Answer from the drawing. Dimensions are ordinates in mm from the lowest x, y and z of the part. A direction names the side the tool comes from. Coordinates: 2 decimals unless noted, no trailing zeros. Order: outer loops, then holes, each group sorted by start corner. A loop starts at its lowest first (then second) coordinate and runs counter-clockwise, first axis right, second up. Notation, with made-up numbers: (-31, 62) - (-18, 62) arc R27 cw to (-18, 96) - close; hole circle Ø2 at (-12.5, -5.5). An arc over 180 degrees is marked (long way). One line per item, written item: value. Start each with the question number.
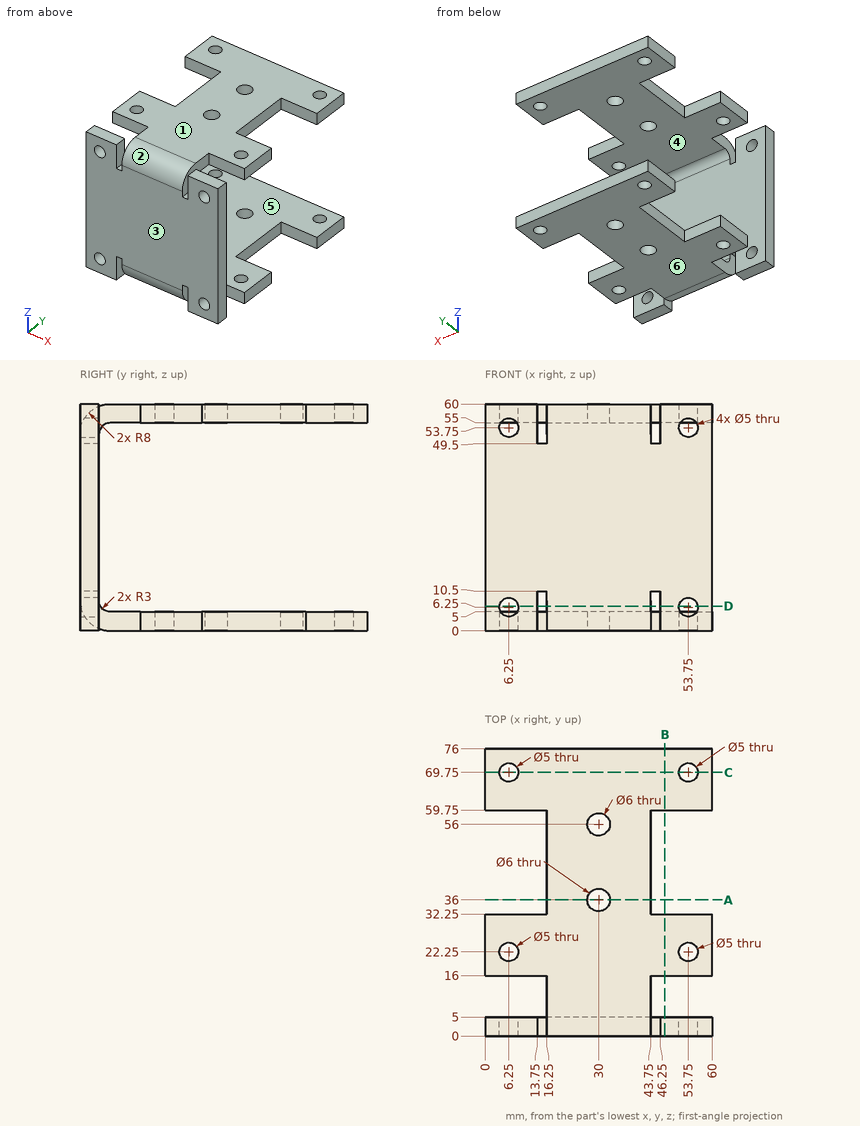
(1) The part is cut by section B-B on x = 47.5. Determine the outline of the cut face in (y, z).
(2) For the marked faces 1 and 2, determine the directions among +Z, -Z, +X, -X, +Y, -Y from which every point of the face is accessible in a straight line to the end or side of a thin tool.
(3) Flat-ended cylindrical pins translate along their axes: pin 1 Ø8 at (x, z) = (22, 31.5) entering from +Y; pin 2 Ø1.2 at (x, y) = (15.5, 2) entering from -Z; pin 3 Ø2.5 at (y, z) = (43.5, 58.5) entering from +X. Find the tip coordinate at first contact, or state that the pin passes through.
(4) For a pull along Z with two mould halves and no side action, classify the marked faces 3, 4, 5 and 6 as pulls with the +Z half, pulls with the -Z half, needs draft (parallel to the pull), parting line crosses it, or undercut.
(5) The part is cut by section D-D on z = 6.5. Determine the outline of the cut face in (x, y), plus the area to 3 significant figures.
(6) The part is cut by section A-A on y = 36. Determine the outline of the cut face in (x, z).
(7) Consider probe 1 along Z at (x, y) = (6, 3); probe 2 along Y at (x, z) = (6.25, 56.8); probe 3 along Y at (x, z) = (53, 57). Determine where each line is inside the solid, lowest interval first.
(8) The part is cut by section C-C on y = 69.75. Determine the outline of the cut face in (x, z), plus the area to 3 significant figures.
Completed:
1. outline: (0, 0) - (5, 0) - (5, 60) - (0, 60) - close; (16, 0) - (32.25, 0) - (32.25, 5) - (16, 5) - close; (16, 55) - (32.25, 55) - (32.25, 60) - (16, 60) - close; (59.75, 0) - (76, 0) - (76, 5) - (59.75, 5) - close; (59.75, 55) - (76, 55) - (76, 60) - (59.75, 60) - close
2. face 1: +Z, +X, -X, +Y, -Y
2. face 2: +Z, -Y
3. pin 1: stops at y = 5
3. pin 2: stops at z = 10.5
3. pin 3: stops at x = 43.75
4. face 3: needs draft
4. face 4: undercut
4. face 5: undercut
4. face 6: pulls with the -Z half
5. outline: (0, 0) - (3.76, 0) - (3.76, 5) - (0, 5) - close; (8.74, 0) - (13.75, 0) - (13.75, 5) - (8.74, 5) - close; (16.25, 0.14) - (43.75, 0.14) - (43.75, 5.4) - (16.25, 5.4) - close; (46.25, 0) - (51.26, 0) - (51.26, 5) - (46.25, 5) - close; (56.24, 0) - (60, 0) - (60, 5) - (56.24, 5) - close
5. area: 232 mm2
6. outline: (16.25, 0) - (27, 0) - (27, 5) - (16.25, 5) - close; (16.25, 55) - (27, 55) - (27, 60) - (16.25, 60) - close; (33, 0) - (43.75, 0) - (43.75, 5) - (33, 5) - close; (33, 55) - (43.75, 55) - (43.75, 60) - (33, 60) - close
7. probe 1: z = 0 to 3.76, 8.74 to 51.26, 56.24 to 60
7. probe 2: y = 0 to 5, 16 to 19.75, 24.75 to 32.25, 59.75 to 67.25, 72.25 to 76
7. probe 3: y = 0 to 5, 16 to 19.87, 24.63 to 32.25, 59.75 to 67.37, 72.13 to 76
8. outline: (0, 0) - (3.75, 0) - (3.75, 5) - (0, 5) - close; (0, 55) - (3.75, 55) - (3.75, 60) - (0, 60) - close; (8.75, 0) - (51.25, 0) - (51.25, 5) - (8.75, 5) - close; (8.75, 55) - (51.25, 55) - (51.25, 60) - (8.75, 60) - close; (56.25, 0) - (60, 0) - (60, 5) - (56.25, 5) - close; (56.25, 55) - (60, 55) - (60, 60) - (56.25, 60) - close
8. area: 500 mm2
